Verification items for the finished model (mm, model axes). Face numbers are marked on the shaded views. A direction names the side the tool comes from. Round coordinates to 2 decimals unless told otherwise and drop trailing zeros. Loops run counter-clockwise (first coordinate to the right, second up) from the corner with the lowest first, then second, coordinate; pieces in that order, holes last. Notation, with made-up numbers: (-29.75, 30) - (11.25, 30) arc R23 ccw to (11.25, 69) - close; hole circle Ø7 at (-9, 70.5). An arc over 180 degrees is marked (long way). Use CSV: the item, a comma, the result in double quotes.
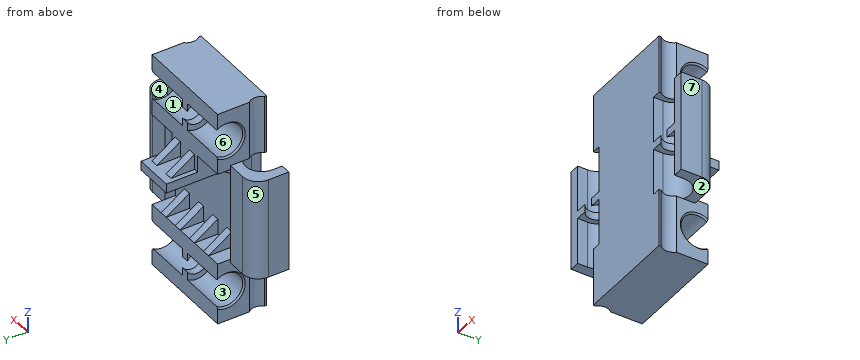
```python
from build123d import *

# Parameters (mm, degrees)
SKETCH_1_W           = 65
SKETCH_1_H           = 140
EXTRUDE_1_DEPTH      = 31.5
SKETCH_2_R           = 10.75
CUT_EXTRUDE_1_DEPTH  = 30
CUT_EXTRUDE_START    = -30
SKETCH_3_R           = 10.75
CUT_EXTRUDE_2_DEPTH  = 30
CHAMFER_1_SIZE       = 1
CHAMFER_2_SIZE       = 1
SKETCH_4_W           = 25
SKETCH_4_H           = 6
EXTRUDE_2_DEPTH      = 20
EXTRUDE_4_DEPTH      = 2.5
EXTRUDE_5_DEPTH      = 2.5
CUT_EXTRUDE_3_DEPTH  = 15
EXTRUDE_6_DEPTH      = 2.5
EXTRUDE_7_DEPTH      = 2.5
EXTRUDE_8_DEPTH      = 2.5
EXTRUDE_9_DEPTH      = 2.5
EXTRUDE_10_DEPTH     = 5
EXTRUDE_11_DEPTH     = 5
SKETCH_18_R          = 7
CUT_EXTRUDE_7_DEPTH  = 94.686978818
SKETCH_19_W          = 65.000437226
SKETCH_19_H          = 23.25
EXTRUDE_12_DEPTH     = 22
SKETCH_20_W          = 65.000437226
SKETCH_20_H          = 23.25
EXTRUDE_13_DEPTH     = 22
CUT_EXTRUDE_8_DEPTH  = 30
SKETCH_22_R          = 7
CUT_EXTRUDE_9_DEPTH  = 159.815931191
CUT_EXTRUDE_10_DEPTH = 30
FILLET_7_R           = 10


with BuildPart() as part:
    # 草图1 → 凸台-拉伸1 (new body)
    with BuildSketch(Plane(origin=(0, 0, 0), x_dir=(1, 0, 0), z_dir=(0, 1, 0))):
        Rectangle(SKETCH_1_W, SKETCH_1_H)
    extrude(amount=EXTRUDE_1_DEPTH)

    # 草图2 → 切除-拉伸1 (cut)
    with BuildSketch(Plane.ZY.offset(32.5)):
        with Locations((-50, 25.5)):
            Circle(SKETCH_2_R)
        with Locations((50, 25.5)):
            Circle(SKETCH_2_R)
    extrude(amount=-CUT_EXTRUDE_1_DEPTH, mode=Mode.SUBTRACT)

    # 草图3 → 切除-拉伸2 (cut)
    with BuildSketch(Plane(origin=(32.5, 0, 0), x_dir=(0, 0, -1), z_dir=(1, 0, 0)).offset(CUT_EXTRUDE_START)):
        with Locations((-50, 25.5)):
            Circle(SKETCH_3_R)
        with Locations((50, 25.5)):
            Circle(SKETCH_3_R)
    extrude(amount=CUT_EXTRUDE_2_DEPTH, mode=Mode.SUBTRACT)

    # 倒角1
    chamfer_1_edges = [part.edges().sort_by_distance(p)[0] for p in [
        (32.5, 14.75, 50),
    ]]
    chamfer(chamfer_1_edges, length=CHAMFER_1_SIZE)

    # 倒角2
    chamfer_2_edges = [part.edges().sort_by_distance(p)[0] for p in [
        (-32.5, 14.75, -50),
        (-32.5, 14.75, 50),
        (32.5, 14.75, -50),
    ]]
    chamfer(chamfer_2_edges, length=CHAMFER_2_SIZE)

    # 草图4 → 凸台-拉伸2 (add)
    with BuildSketch(Plane(origin=(0, 31.5, 0), x_dir=(1, 0, 0), z_dir=(0, 1, 0))):
        with Locations((0, -16.15)):
            Rectangle(SKETCH_4_W, SKETCH_4_H)
    extrude(amount=EXTRUDE_2_DEPTH)

    # 草图7 → 凸台-拉伸4 (add, symmetric)
    with BuildSketch(Plane(origin=(7, 0, 0), x_dir=(0, 0, -1), z_dir=(1, 0, 0))):
        Polygon((-19.15, 46.5), (-19.15, 31.5), (-29.15, 31.5), align=None)
    extrude(amount=EXTRUDE_4_DEPTH, both=True)

    # 草图8 → 凸台-拉伸5 (add, symmetric)
    with BuildSketch(Plane(origin=(-7, 0, 0), x_dir=(0, 0, -1), z_dir=(1, 0, 0))):
        Polygon((-19.15, 46.5), (-19.15, 31.5), (-29.15, 31.5), align=None)
    extrude(amount=EXTRUDE_5_DEPTH, both=True)

    # 草图9 → 切除-拉伸3 (cut)
    with BuildSketch(Plane(origin=(0, 31.5, 0), x_dir=(1, 0, 0), z_dir=(0, 1, 0))):
        Polygon((-32.5, 30.000218613), (32.5, 30.000218613), (32.5, -13.15), (32.5, -30.000218613), (12.5, -30.000218613), (12.5, -13.15), (-12.5, -13.15), (-12.5, -30.000218613), (-32.5, -30.000218613), (-32.5, -13.15), align=None)
    extrude(amount=-CUT_EXTRUDE_3_DEPTH, mode=Mode.SUBTRACT)

    # 草图11 → 凸台-拉伸6 (add, symmetric)
    with BuildSketch(Plane(origin=(7, 0, 0), x_dir=(0, 0, -1), z_dir=(1, 0, 0))):
        Polygon((30.000218613, 31.5), (30.000218613, 16.5), (20.000218613, 16.5), align=None)
    extrude(amount=EXTRUDE_6_DEPTH, both=True)

    # 草图13 → 凸台-拉伸7 (add, symmetric)
    with BuildSketch(Plane(origin=(21, 0, 0), x_dir=(0, 0, -1), z_dir=(1, 0, 0))):
        Polygon((30.000218613, 31.5), (30.000218613, 16.5), (20.000218613, 16.5), align=None)
    extrude(amount=EXTRUDE_7_DEPTH, both=True)

    # 草图12 → 凸台-拉伸8 (add, symmetric)
    with BuildSketch(Plane(origin=(-7, 0, 0), x_dir=(0, 0, -1), z_dir=(1, 0, 0))):
        Polygon((30.000218613, 31.5), (30.000218613, 16.5), (20.000218613, 16.5), align=None)
    extrude(amount=EXTRUDE_8_DEPTH, both=True)

    # 草图14 → 凸台-拉伸9 (add, symmetric)
    with BuildSketch(Plane(origin=(-21, 0, 0), x_dir=(0, 0, -1), z_dir=(1, 0, 0))):
        Polygon((30.000218613, 31.5), (30.000218613, 16.5), (20.000218613, 16.5), align=None)
    extrude(amount=EXTRUDE_9_DEPTH, both=True)

    # 草图15 → 凸台-拉伸10 (add)
    with BuildSketch(Plane(origin=(-21, 0, 0), x_dir=(0, 0, -1), z_dir=(1, 0, 0))):
        Polygon((-30.000218613, 31.5), (-30.000218613, 16.5), (-20.000218613, 16.5), align=None)
    extrude(amount=-EXTRUDE_10_DEPTH)

    # 草图16 → 凸台-拉伸11 (add)
    with BuildSketch(Plane(origin=(21, 0, 0), x_dir=(0, 0, -1), z_dir=(1, 0, 0))):
        Polygon((-30.000218613, 31.5), (-30.000218613, 16.5), (-20.000218613, 16.5), align=None)
    extrude(amount=EXTRUDE_11_DEPTH)

    # 草图18 → 切除-拉伸7 (cut, through all)
    with BuildSketch(Plane.ZY.offset(2.5)):
        with Locations((50, 25.5)):
            Circle(SKETCH_18_R)
        with Locations((-50, 25.5)):
            Circle(SKETCH_18_R)
    extrude(amount=-CUT_EXTRUDE_7_DEPTH, mode=Mode.SUBTRACT)

    # 草图19 → 凸台-拉伸12 (add)
    with BuildSketch(Plane(origin=(32.5, 0, 0), x_dir=(0, 0, -1), z_dir=(1, 0, 0))):
        with Locations((0, 11.625)):
            Rectangle(SKETCH_19_W, SKETCH_19_H)
    extrude(amount=EXTRUDE_12_DEPTH)

    # 草图20 → 凸台-拉伸13 (add)
    with BuildSketch(Plane.ZY.offset(32.5)):
        with Locations((0, 11.625)):
            Rectangle(SKETCH_20_W, SKETCH_20_H)
    extrude(amount=EXTRUDE_13_DEPTH)

    # 草图21 → 切除-拉伸8 (cut)
    with BuildSketch(Plane.XY.offset(32.500218613)):
        with BuildLine():
            Line((-48, 6.25), (-48, 0))
            Line((-48, 0), (-27, 0))
            Line((-27, 0), (-27, 6.25))
            ThreePointArc((-27, 6.25), (-37.5, 16.75), (-48, 6.25))
        make_face()
        with BuildLine():
            Line((27, 6.25), (27, 0))
            Line((27, 0), (48, 0))
            Line((48, 0), (48, 6.25))
            ThreePointArc((48, 6.25), (37.5, 16.75), (27, 6.25))
        make_face()
    extrude(amount=-CUT_EXTRUDE_8_DEPTH, mode=Mode.SUBTRACT)

    # 草图22 → 切除-拉伸9 (cut, through all)
    with BuildSketch(Plane.XY.offset(70)):
        with Locations((-37.5, 6.25)):
            Circle(SKETCH_22_R)
        with Locations((37.5, 6.25)):
            Circle(SKETCH_22_R)
    extrude(amount=-CUT_EXTRUDE_9_DEPTH, mode=Mode.SUBTRACT)

    # 草图23 → 切除-拉伸10 (cut)
    with BuildSketch(Plane(origin=(0, 0, -32.500218613), x_dir=(-1, 0, 0), z_dir=(0, 0, -1)).offset(CUT_EXTRUDE_START)):
        with BuildLine():
            Line((-48, 6.25), (-48, 0))
            Line((-48, 0), (-27, 0))
            Line((-27, 0), (-27, 6.25))
            ThreePointArc((-27, 6.25), (-37.5, 16.75), (-48, 6.25))
        make_face()
        with BuildLine():
            Line((48, 6.25), (48, 0))
            Line((48, 0), (27, 0))
            Line((27, 0), (27, 6.25))
            ThreePointArc((27, 6.25), (37.5, 16.75), (48, 6.25))
        make_face()
    extrude(amount=CUT_EXTRUDE_10_DEPTH, mode=Mode.SUBTRACT)

    # 圆角7
    fillet_7_edges = [part.edges().sort_by_distance(p)[0] for p in [
        (54.5, 23.25, 0),
        (-54.5, 23.25, 0),
    ]]
    fillet(fillet_7_edges, radius=FILLET_7_R)


solid = part.part
```
1) Mould release check, pull along Y, two halves, no side actions. Record for the marked faces 5, 6 and 7: +Y half, -Y half, draft (parallel to the pull), parting line (faces both ways), or undercut.
Returned:
face 5,"+Y half"
face 6,"undercut"
face 7,"draft"
2) Access from +Z, -Z, +X, -X, +Y, -Y to the whole of each face (thin tool, end or side, straight path). Record for the marked faces 1, 2, 3 and 4.
Returned:
face 1,"+X"
face 2,"-Z, +X, +Y, -Y"
face 3,"-X"
face 4,"+Z, +X, +Y, -Y"
3) Cross-section at A-A, the plane y = 37.5. Record the cut outline in (x, z), then the cut area to 3 significant figures.
Returned:
outline,"(-12.5, 13.15) - (12.5, 13.15) - (12.5, 19.15) - (9.5, 19.15) - (9.5, 25.15) - (4.5, 25.15) - (4.5, 19.15) - (-4.5, 19.15) - (-4.5, 25.15) - (-9.5, 25.15) - (-9.5, 19.15) - (-12.5, 19.15) - close"
area,"210 mm²"
4) Thickness scan on probe 1 along Z at (x, y) = (17.25, 25.5); probe 2 along X at (y, z) = (26, 29); probe 3 along Y at (x, z) = (-15, -50). Record the ranges inside material, lowest first. Write a range as [from, to].
Returned:
probe 1,"z = [-70, -60.75], [-39.25, -30], [30, 39.25], [60.75, 70]"
probe 2,"x = [-26, -21], [-12.5, 12.5], [21, 26]"
probe 3,"y = [0, 14.75]"
5) Cross-section at C-C, the plane x = -37.5. Record the cut outline in (y, z), then the cut area to 3 significant figures.
Returned:
outline,"(13.25, -2.5) - (16.75, -2.5) - (16.75, -32.5) - (23.25, -32.5) - (23.25, 32.5) - (16.75, 32.5) - (16.75, 2.5) - (13.25, 2.5) - close"
area,"440 mm²"
6) Cross-section at B-B, the plane z = -50. Record the cut outline in (x, y), then the cut area to 3 significant figures.
Returned:
outline,"(-32.5, 0) - (32.5, 0) - (32.5, 1.35) arc R7 cw to (32.5, 11.15) - (32.5, 13.75) - (31.5, 14.75) - (2.5, 14.75) - (2.5, 18.5) - (-2.5, 18.5) - (-2.5, 14.75) - (-31.5, 14.75) - (-32.5, 13.75) - (-32.5, 11.15) arc R7 cw to (-32.5, 1.35) - close"
area,"950 mm²"
7) Gauge pin test, flat ends, axial feed: pin 1 Ø10 at (y, z) = (17, 47.5) entering from -X; pin 2 Ø8 at (x, y) = (-43, 11.5) entering from +Z; pin 3 Ø16.5 at (y, z) = (22.5, -49) entering from -X. Record the tip position at first contact, or that the pin passes through.
Returned:
pin 1,"stops at x = -32.5"
pin 2,"stops at z = 32.5"
pin 3,"stops at x = -32.16"
8) Cross-section at D-D, the plane y = 21. Count the separate pieces of the cut face and the enclosed holes in it, then the cut area to 3 significant figures.
Returned:
separate pieces,"3"
enclosed holes,"1"
area,"5,760 mm²"
